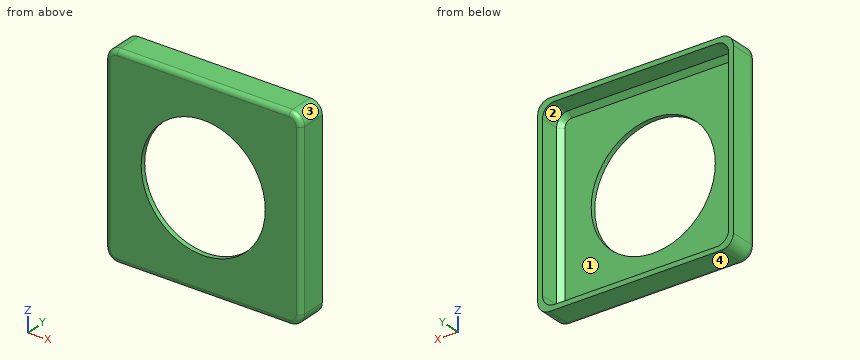
Autodesk Inventor part; units mm, degrees
ref_plane "YZ Plane" through (0, 0, 0) normal (1, 0, 0) x (0, 1, 0)
ref_plane "XZ Plane" through (0, 0, 0) normal (0, 1, 0) x (-1, 0, 0)
ref_plane "XY Plane" through (0, 0, 0) normal (0, 0, 1) x (1, 0, 0)
sketch "Sketch1" plane through (0, 0, 0) normal (0, 1, 0) x (-1, 0, 0)
  line L0 (28.931, 30.3524) -> (-43.069, 30.3524)
  line L1 (-48.069, 25.3524) -> (-48.069, -51.6476)
  line L2 (-43.069, -51.6476) -> (33.931, -51.6476)
  line L3 (33.931, -46.6476) -> (33.931, 30.3524)
  arc A0 (-48.069, -46.6476) -> (-43.069, -51.6476) centre (-43.069, -46.6476) ccw
  line L4 (-46.069, 28.3524) -> (26.931, 28.3524)
  line L5 (31.931, 23.3524) -> (31.931, -44.6476)
  line L6 (31.931, -49.6476) -> (-46.069, -49.6476)
  line L7 (-46.069, -44.6476) -> (-46.069, 23.3524)
  arc A1 (-38.6778, 27.7435) -> (-45.4601, 20.9612) centre (-41.069, 23.3524) ccw
  arc A2 (24.5399, -49.0388) -> (31.3222, -42.2565) centre (26.931, -44.6476) ccw
  arc A3 (31.3222, 20.9612) -> (24.5399, 27.7435) centre (26.931, 23.3524) ccw
  arc A4 (-45.4601, -42.2565) -> (-38.6778, -49.0388) centre (-41.069, -44.6476) ccw
  arc A5 (33.931, 25.3524) -> (28.931, 30.3524) centre (28.931, 25.3524) ccw
  arc A6 (-46.069, 21.3524) -> (-45.4601, 20.9612) centre (-43.069, 25.3524) ccw
  arc A7 (-43.069, 30.3524) -> (-48.069, 25.3524) centre (-43.069, 25.3524) ccw
  arc A8 (28.931, -51.6476) -> (33.931, -46.6476) centre (28.931, -46.6476) ccw
  point P0 (0, 0)
  point P1 (-41.069, -49.6476)
  point P2 (26.931, -49.6476)
  point P3 (-41.069, 28.3524)
  dimension "d0" = 82
  dimension "d1" = 82
  dimension "d3" = 10
  dimension "d7" = 78
  dimension "d8" = 78
  dimension "d9" = 2
  dimension "d10" = 2
  dimension "d11" = 10
  dimension "d12" = 10
  dimension "d13" = 10
  dimension "d14" = 10
extrude "Extrusion1" add sketch "Sketch1" along normal blind 2 contours L4 A3 L5 A2 L6 A4 L7 A6 A1
extrude "Extrusion2" add sketch "Sketch1" along normal blind 15
sketch "Sketch2" plane through (0, 0, 0) normal (0, -1, 0) x (1, 0, 0)
  line L0 (48.069, 25.3524) -> (48.069, -46.6476)
  arc A0 (48.069, 25.3524) -> (43.069, 30.3524) centre (43.069, 25.3524) ccw
  line L1 (-28.931, 30.3524) -> (43.069, 30.3524)
  arc A1 (-28.931, 30.3524) -> (-33.931, 25.3524) centre (-28.931, 25.3524) ccw
  line L2 (-33.931, -46.6476) -> (-33.931, 25.3524)
  arc A2 (-33.931, -46.6476) -> (-28.931, -51.6476) centre (-28.931, -46.6476) ccw
  line L3 (43.069, -51.6476) -> (-28.931, -51.6476)
  arc A3 (43.069, -51.6476) -> (48.069, -46.6476) centre (43.069, -46.6476) ccw
  arc A4 (45.4601, 20.9612) -> (46.069, 21.3524) centre (43.069, 25.3524) ccw
  arc A5 (45.4601, 20.9612) -> (46.069, 23.3524) centre (41.069, 23.3524) ccw
  line L4 (46.069, 21.3524) -> (46.069, 23.3524)
  circle A6 centre (7.069, -10.6476) radius 26
  point P0 (0, 0)
  dimension "d19" = 52
extrude "Extrusion3" cut sketch "Sketch2" along normal mid plane 15 contours A6
sketch "Sketch3" plane through (0, 15, 0) normal (0, 1, 0) x (1, 0, 0)
  line L0 (48.069, -25.3524) -> (48.069, 46.6476)
  arc A0 (48.069, 46.6476) -> (43.069, 51.6476) centre (43.069, 46.6476) ccw
  line L1 (43.069, 51.6476) -> (-28.931, 51.6476)
  arc A1 (-28.931, 51.6476) -> (-33.931, 46.6476) centre (-28.931, 46.6476) ccw
  line L2 (-33.931, 46.6476) -> (-33.931, -25.3524)
  arc A2 (-33.931, -25.3524) -> (-28.931, -30.3524) centre (-28.931, -25.3524) ccw
  line L3 (-28.931, -30.3524) -> (43.069, -30.3524)
  arc A3 (43.069, -30.3524) -> (48.069, -25.3524) centre (43.069, -25.3524) ccw
  arc A4 (46.069, 44.6476) -> (41.069, 49.6476) centre (41.069, 44.6476) ccw
  line L4 (46.069, 44.6476) -> (46.069, -23.3524)
  arc A5 (41.069, -28.3524) -> (46.069, -23.3524) centre (41.069, -23.3524) ccw
  line L5 (41.069, -28.3524) -> (-26.931, -28.3524)
  arc A6 (-31.931, -23.3524) -> (-26.931, -28.3524) centre (-26.931, -23.3524) ccw
  line L6 (-31.931, -23.3524) -> (-31.931, 44.6476)
  arc A7 (-26.931, 49.6476) -> (-31.931, 44.6476) centre (-26.931, 44.6476) ccw
  line L7 (-26.931, 49.6476) -> (41.069, 49.6476)
  point P0 (0, 0)
extrude "Extrusion4" cut sketch "Sketch3" against normal blind 3
fillet "Fillet1" radius 2 8 edges at (7.069, 0, -51.6476) (-32.4666, 0, -50.1832) (-33.931, 0, -10.6476) (-32.4666, 0, 28.8879) (7.069, 0, 30.3524) (46.6045, 0, 28.8879) (48.069, 0, -10.6476) (46.6045, 0, -50.1832)
sketch "Sketch4" plane through (0, 0, 0) normal (0, -1, 0) x (1, 0, 0)
  line L0 (46.069, 21.3524) -> (46.069, -46.6476)
  arc A0 (45.4601, 20.9612) -> (46.069, 21.3524) centre (43.069, 25.3524) ccw
  arc A1 (45.4601, 20.9612) -> (46.069, 23.3524) centre (41.069, 23.3524) ccw
  line L1 (46.069, 25.3524) -> (46.069, 23.3524)
  arc A2 (46.069, 25.3524) -> (43.069, 28.3524) centre (43.069, 25.3524) ccw
  line L2 (-28.931, 28.3524) -> (43.069, 28.3524)
  arc A3 (-28.931, 28.3524) -> (-31.931, 25.3524) centre (-28.931, 25.3524) ccw
  line L3 (-31.931, -46.6476) -> (-31.931, 25.3524)
  arc A4 (-31.931, -46.6476) -> (-28.931, -49.6476) centre (-28.931, -46.6476) ccw
  line L4 (43.069, -49.6476) -> (-28.931, -49.6476)
  arc A5 (43.069, -49.6476) -> (46.069, -46.6476) centre (43.069, -46.6476) ccw
  circle A6 centre (7.069, -10.6476) radius 26
  line L5 (46.069, 23.3524) -> (46.069, -44.6476)
  line L6 (46.069, 21.3524) -> (46.069, 23.3524)
  point P0 (0, 0)
extrude "Extrusion5" add sketch "Sketch4" against normal blind 2 contours A0 A1 L5
chamfer "Chamfer1" distance 2 angle 45 8 edges at (46.069, 2, -10.6476) (44.6045, 2, 26.8879) (7.069, 2, 28.3524) (-30.4666, 2, 26.8879) (-31.931, 2, -10.6476) (-30.4666, 2, -48.1832) (7.069, 2, -49.6476) (44.6045, 2, -48.1832)
properties part number "controler_03"
Model file for the job. Use its own axes, mm. Face numbers are marked on the shaded views. Coordinates: 2 decimals unless noted, no trailing zeros. Loops run counter-clockwise (first coordinate to the right, second up) from the corner with the lowest first, then second, coordinate; pieces in that order, holes last. Notation, with made-up numbers: (22, -17) - (75, -17) arc R26 cw to (75, -1) - close; hole circle Ø9 at (-31, 23). An arc over 180 degrees is marked (long way). Write item = value, one per line. Start each with the question number.
Item 1: Saw through at B-B, the plane z = -15.5. List the corners of the cut face in (x, y).
Item 2: Pull direction X, two halves, no side cores. Call the marked faces 1, 2, 3 and 4: +X half, -X half, draft (parallel to the pull), parting line (faces both ways), or undercut.
Item 3: Saw through at A-A, the plane x = 7. List the corners of the cut face in (y, z), then the cut area to 3 significant figures.
Item 4: Drop a flat-ended pin along its axis: pin 1 Ø6 at (x, z) = (23, -28.5) entering from +Y. Give the stop position or say it passes through.
Item 5: Saw through at C-C, the plane y = 3. List the corners of the cut face in (x, z), then the cut area to 3 significant figures.
Item 6: Wall check: probe 1 along X at (y, z) = (4, 6); probe 2 along Z at (x, y) = (34, 9); probe 3 along Z at (x, y) = (41.5, 9.5). Give the ranges that are in metal, low to high. Write a range as [from, to].
Item 7: Saw through at D-D, the plane y = 9. List the corners of the cut face in (x, z).
Answers:
q1.outline = (-33.93, 2) arc R2 ccw to (-31.93, 0) - (-18.47, 0) - (-18.47, 2) - (-29.93, 2) - (-31.93, 4) - (-31.93, 12) - (-33.93, 12) - close; (32.61, 0) - (46.07, 0) arc R2 ccw to (48.07, 2) - (48.07, 12) - (46.07, 12) - (46.07, 4) - (44.07, 2) - (32.61, 2) - close
q2.face_1 = undercut
q2.face_2 = undercut
q2.face_3 = +X half
q2.face_4 = draft
q3.outline = (0, -49.65) arc R2 ccw to (2, -51.65) - (12, -51.65) - (12, -49.65) - (4, -49.65) - (2, -47.65) - (2, -36.65) - (0, -36.65) - close; (0, 15.35) - (2, 15.35) - (2, 26.35) - (4, 28.35) - (12, 28.35) - (12, 30.35) - (2, 30.35) arc R2 ccw to (0, 28.35) - close
q3.area = 102 mm2
q4.pin_1 = 2
q5.outline = (-33.93, -46.65) arc R5 ccw to (-28.93, -51.65) - (43.07, -51.65) arc R5 ccw to (48.07, -46.65) - (48.07, 25.35) arc R5 ccw to (43.07, 30.35) - (-28.93, 30.35) arc R5 ccw to (-33.93, 25.35) - close; hole (-30.93, -44.65) arc R4 ccw to (-26.93, -48.65) - (41.07, -48.65) arc R4 ccw to (45.07, -44.65) - (45.07, 23.35) arc R4 ccw to (41.07, 27.35) - (-26.93, 27.35) arc R4 ccw to (-30.93, 23.35) - close
q5.area = 940 mm2
q6.probe_1 = [-33.93, -31.93], [46.07, 48.07]
q6.probe_2 = [-51.65, -49.65], [28.35, 30.35]
q6.probe_3 = [-51.65, -49.63], [28.33, 30.35]
q7.outline = (-33.93, -46.65) arc R5 ccw to (-28.93, -51.65) - (43.07, -51.65) arc R5 ccw to (48.07, -46.65) - (48.07, 25.35) arc R5 ccw to (43.07, 30.35) - (-28.93, 30.35) arc R5 ccw to (-33.93, 25.35) - close; hole (-31.93, -44.65) arc R5 ccw to (-26.93, -49.65) - (41.07, -49.65) arc R5 ccw to (46.07, -44.65) - (46.07, 23.35) arc R5 ccw to (41.07, 28.35) - (-26.93, 28.35) arc R5 ccw to (-31.93, 23.35) - close
